Part model, mm, in its own coordinate system. Face numbers are marked on the shaded views. A direction names the side the tool comes from. Round coordinates to 2 decimals unless told otherwise and drop trailing zeros. Loops run counter-clockwise (first coordinate to the right, second up) from the corner with the lowest first, then second, coordinate; pieces in that order, holes last. Notation, with made-up numbers: M 26,-19 L 80,-19 A6 ccw 80,-10 Z; hole C 33,49.5 d9. An arc over 180 degrees is marked long. Put each result on its own line as item: value. Start each with the question number.
1) Slice it at D-D on z = 35. Give the cut face in (x, y).
2) Slice it at B-B on x = 7.75. Give the cut face in (y, z), then the cut area to 3 significant figures.
3) Probe line 1 along Z through (x, y) = (8.4, 130); line 2 along Z through (x, y) = (6.25, 68.5); line 3 along Z through (x, y) = (3.25, 113.5). List the from-to ranges inside material, lowest first.
4) Slice it at A-A on z = -20. Give the cut face in (x, y), then the cut area to 4 significant figures.
5) Slice it at C-C on y = 5. Give the cut face in (x, z), then the cut area to 3 significant figures.
6) Pull direction Z, two halves, no side cores. Call the marked faces 3, 4 and 5: +Z half, -Z half, draft (parallel to the pull), parting line (faces both ways), or undercut.
7) Drop flat-ended pins along their axis: pin 1 Ø3 at (y, z) = (4.5, 19.5) entering from +X; pin 2 Ø2 at (x, y) = (3.5, 26.5) entering from -Z; pin 3 Ø3 at (x, y) = (2, 133) entering from +Z. Give the stop position or say it passes through.
8) Which spindle directions (+Z, -Z, +X, -X, +Y, -Y) get a long thin tool onto all of the face, cutting with end or side? Do the marked faces 1 and 2. Say none if no direction does.
```python
from build123d import *

# Parameters (mm, degrees)
BOSS_EXTRUDE1_DEPTH = 10
CUT_EXTRUDE1_DEPTH  = 6
SKETCH4_R           = 1.65
CUT_EXTRUDE2_DEPTH  = 11
SKETCH5_R           = 3
CUT_EXTRUDE3_DEPTH  = 5
SKETCH6_R           = 1.5
CUT_EXTRUDE4_DEPTH  = 5
CUT_EXTRUDE6_DEPTH  = 11


with BuildPart() as part:
    # Sketch2 → Boss-Extrude1 (new body)
    with BuildSketch(Plane(origin=(0, 0, 0), x_dir=(0, 0, -1), z_dir=(1, 0, 0))):
        with BuildLine():
            Line((40, 0), (-40, 0))
            Line((-40, 0), (-15, 130))
            ThreePointArc((-15, 130), (0, 145), (15, 130))
            Line((15, 130), (40, 0))
        make_face()
    extrude(amount=BOSS_EXTRUDE1_DEPTH)

    # Sketch3 → Cut-Extrude1 (cut)
    with BuildSketch(Plane.ZY):
        with BuildLine():
            Line((-10, 130), (-10, 151.126505972))
            Line((-10, 151.126505972), (10, 151.126505972))
            Line((10, 151.126505972), (10, 130))
            ThreePointArc((10, 130), (0, 120), (-10, 130))
        make_face()
    extrude(amount=-CUT_EXTRUDE1_DEPTH, mode=Mode.SUBTRACT)

    # Sketch4 → Cut-Extrude2 (cut, through all)
    with BuildSketch(Plane.ZY):
        with Locations((20, 5)):
            Circle(SKETCH4_R)
        with Locations((-20, 5)):
            Circle(SKETCH4_R)
    extrude(amount=-CUT_EXTRUDE2_DEPTH, mode=Mode.SUBTRACT)

    # Sketch5 → Cut-Extrude3 (cut)
    with BuildSketch(Plane(origin=(10, 0, 0), x_dir=(0, 0, -1), z_dir=(1, 0, 0))):
        with Locations((-20, 5)):
            Circle(SKETCH5_R)
        with Locations((20, 5)):
            Circle(SKETCH5_R)
    extrude(amount=-CUT_EXTRUDE3_DEPTH, mode=Mode.SUBTRACT)

    # Sketch6 → Cut-Extrude4 (cut, through all)
    with BuildSketch(Plane.ZY.offset(-6)):
        with Locations((0, 130)):
            Circle(SKETCH6_R)
    extrude(amount=-CUT_EXTRUDE4_DEPTH, mode=Mode.SUBTRACT)

    # Sketch7 → Cut-Extrude6 (cut, through all)
    with BuildSketch(Plane.ZY):
        Polygon((0, 102.094381641), (-15.787381085, 20), (15.787381085, 20), align=None)
    extrude(amount=-CUT_EXTRUDE6_DEPTH, mode=Mode.SUBTRACT)


solid = part.part
```
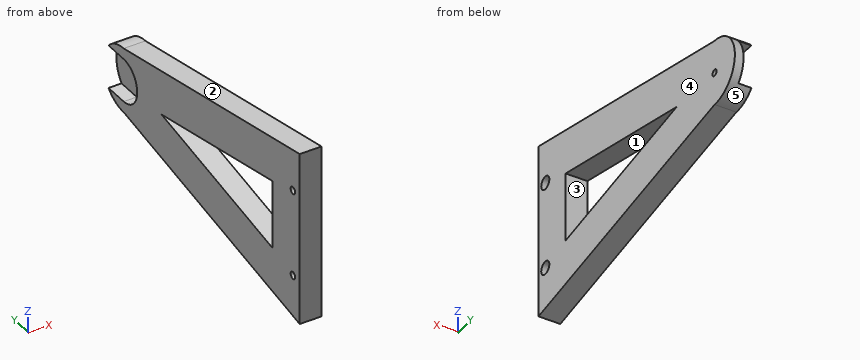
Recorded:
1. outline: M 0,0 L 10,0 L 10,26 L 0,26 Z
2. outline: M 0,-40 L 130,-15 A15 ccw 130,15 L 0,40 Z; hole C 5,-20 d6; hole C 5,20 d6; hole M 20,-15.79 L 102.09,0 L 20,15.79 Z; hole C 130,0 d3
2. area: 6,140 mm2
3. line 1: z = -15 to -1.5, 1.5 to 15
3. line 2: z = -26.83 to -6.46, 6.46 to 26.83
3. line 3: z = -18.17 to 18.17
4. outline: M 0,0 L 10,0 L 10,2 L 5,2 L 5,3.35 L 0,3.35 Z; M 0,6.65 L 5,6.65 L 5,8 L 10,8 L 10,104 L 0,104 Z
4. area: 993.5 mm2
5. outline: M 0,-39.04 L 10,-39.04 L 10,-23 L 5,-23 L 5,-21.65 L 0,-21.65 Z; M 0,-18.35 L 5,-18.35 L 5,-17 L 10,-17 L 10,17 L 5,17 L 5,18.35 L 0,18.35 Z; M 0,21.65 L 5,21.65 L 5,23 L 10,23 L 10,39.04 L 0,39.04 Z
5. area: 688 mm2
6. face 3: undercut
6. face 4: draft
6. face 5: parting line
7. pin 1: stops at x = 5
7. pin 2: stops at z = -35.1
7. pin 3: stops at z = 14.92
8. face 1: +X, -X
8. face 2: +Z, +X, -X, +Y
